from build123d import *

# Parameters (mm, degrees)
F0_R     = 40
F0_R_2   = 5
F1_DEPTH = 85
F3_R     = 37.5
F4_DEPTH = 82.5
F5_W     = 5
F5_H     = 2.5
F5_W_2   = 35
F5_H_2   = 5
F6_DEPTH = 50
F8_COUNT = 2


with BuildPart() as f1:
    # F0 (on Top) → F1 (new body)
    with BuildSketch(Plane.XY):
        Circle(F0_R)
        Circle(F0_R_2, mode=Mode.SUBTRACT)
    extrude(amount=F1_DEPTH)

    # F3 (on face) → F4 (cut)
    with BuildSketch(Plane.XY.offset(85)):
        Circle(F3_R)
    extrude(amount=-F4_DEPTH, mode=Mode.SUBTRACT)


with BuildPart() as f6:
    # F5 (on Right) → F6 (new body)
    with BuildSketch(Plane.YZ):
        Polygon((5, 82.5), (5, 80), (40, 80), (40, 85), (5, 85), align=None)
        with Locations((2.5, 81.25)):
            Rectangle(F5_W, F5_H)
        with Locations((-22.5, 82.5)):
            Rectangle(F5_W_2, F5_H_2)
    extrude(amount=F6_DEPTH)


with BuildPart() as f8_1:
    # F8: instance of F6
    add(f6.part.rotate(Axis((0, 0, 42.584691), (0, 0, 1)), 1 * 360 / F8_COUNT))


with BuildPart() as f1_1:
    add(f1.part)

    # F9: cut F6, F8_1
    add(f6.part, mode=Mode.SUBTRACT)
    add(f8_1.part, mode=Mode.SUBTRACT)


solid = f1_1.part
Verification items for the finished model (mm, model axes). A direction names the side the tool comes from. Coordinates: 2 decimals unless noted, no trailing zeros. Order: outer loops, then holes, each group sorted by start corner. A loop starts at its lowest first (then second) coordinate and runs counter-clockwise, first axis right, second up. Notation, with made-up numbers: (5.25, 77.5) -> (36.25, 77.5) arc R15 ccw to (36.25, 82.5) -> close; hole circle Ø2 at (-18, 18). An arc over 180 degrees is marked (long way). Use CSV: the item, a comma, the result in double quotes. Start each with the question number.
Q1. Section check D-D, the plane z = 69.5. Record the cut outline in (x, y), and give its area (3 significant figures).
Q2. Thickness scan on line 1 along Z through (x, y) = (25, 2); line 2 along Z through (x, y) = (-36.5, -11.5); line 3 along Y through (x, z) = (-19.5, 14.5). Record the ranges inside material, lowest first.
Q3. Tool access check on faces 1 (the flat face through (-39, 0, 81)), 2 (the flat face through (38, -5, 82)), 3 (the flat face through (39, 0, 81)). Record the directions out of +Z, -Z, +X, -X, +Y, -Y that give a thin tool (end or side, any length) a straight path to the whole face; none if there is none.
Q4. Section check B-B, the plane y = 2.5. Record the cut outline in (x, z), and give its area (3 significant figures).
Q5. Depth check by flat-ended pin: P1, Ø13, axis at x = 0, y = 0, coming from the +Z side; P2, Ø4, axis at y = 8, z = 28, coming from the -X side; P3, Ø1.3, axis at x = 38, z = 83.5, coming from the -Y side. Enter the tip coordinate at first touch or a pass-through.
Q6. Section check C-C, the plane x = -25. Record the cut outline in (y, z).
Q7. Draft check along X on faces 4 (the flat face through (39, 0, 85)), 5 (the flat face through (8, 1, 2.5)). Enter one of: +X half, -X half, draft (parallel to the pull), parting line (faces both ways), or undercut.
Q8. Section check A-A, the plane x = 0. Record the cut outline in (y, z).
Returned:
1,outline,"circle Ø80 at (0, 0); hole circle Ø75 at (0, 0)"
1,area,"609 mm^2"
2,line 1,"z = 0 to 2.5"
2,line 2,"z = 0 to 80"
2,line 3,"y = -34.92 to -32.03, 32.03 to 34.92"
3,face 1,"-X, -Y"
3,face 2,"+Z, +X, -X, -Y"
3,face 3,"+X, +Y"
4,outline,"(-39.92, 0) -> (-4.33, 0) -> (-4.33, 2.5) -> (-37.42, 2.5) -> (-37.42, 85) -> (-39.92, 85) -> close; (4.33, 0) -> (39.92, 0) -> (39.92, 80) -> (37.42, 80) -> (37.42, 2.5) -> (4.33, 2.5) -> close; (37.42, 82.5) -> (39.92, 82.5) -> (39.92, 85) -> (37.42, 85) -> close"
4,area,"585 mm^2"
5,P1,"stops at z = 2.5"
5,P2,"stops at x = -39.55"
5,P3,"stops at y = -5"
6,outline,"(-31.22, 0) -> (31.22, 0) -> (31.22, 80) -> (27.95, 80) -> (27.95, 2.5) -> (-27.95, 2.5) -> (-27.95, 80) -> (-31.22, 80) -> close"
7,face 4,"draft"
7,face 5,"undercut"
8,outline,"(-40, 0) -> (-5, 0) -> (-5, 2.5) -> (-37.5, 2.5) -> (-37.5, 80) -> (-40, 80) -> close; (5, 0) -> (40, 0) -> (40, 80) -> (37.5, 80) -> (37.5, 2.5) -> (5, 2.5) -> close"
